Answer from the drawing. Dimensions are ordinates in mm from the lowest x, y and z of the part. A direction names the side the tool comes from. Give positions to 0.01 mm unless a question says otherwise; leave off trailing zeros. Write item = value, one per line.
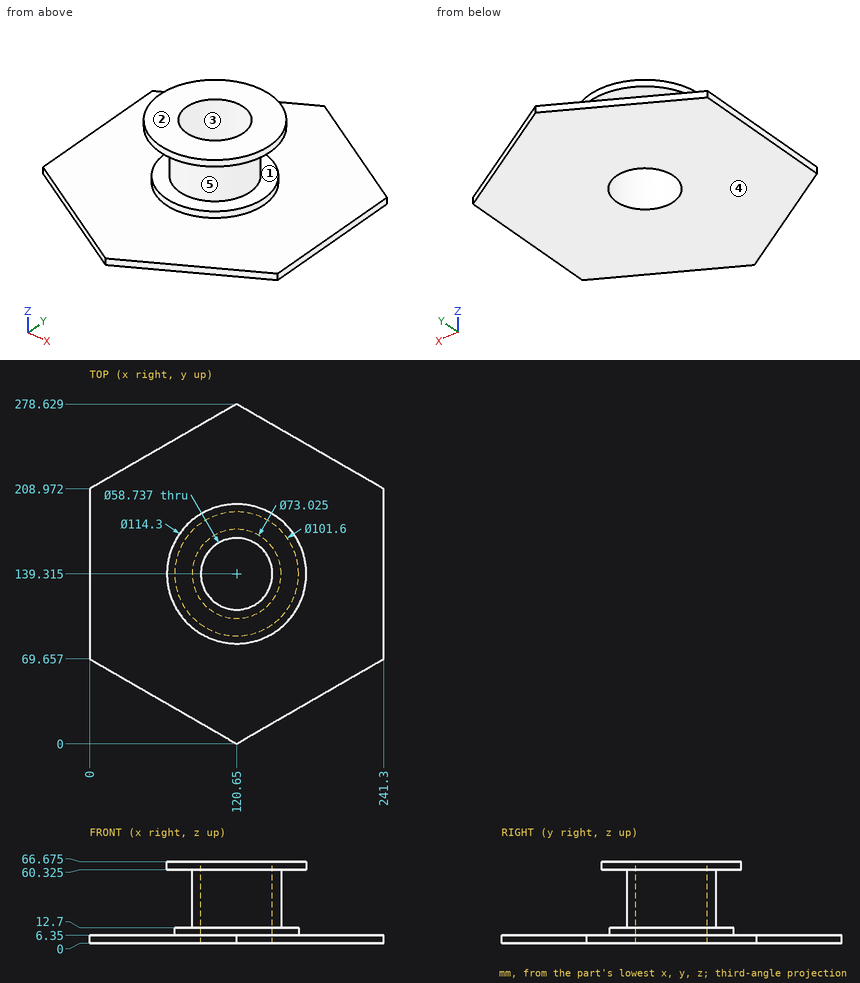
(1) Consider L1, parallel to Z at x = 113.5, y = 183.5 (1 decimal); L2, parallel to Y at x = 120.65, z = 53.5 (1 decimal); L3, parallel to Y at x = 120, z = 34. Determine where each line is inside the solid, lowest interval first.
Checks:
L1 = 0 to 12.7, 60.3 to 66.7
L2 = 102.8 to 109.9, 168.7 to 175.8
L3 = 102.81 to 109.95, 168.68 to 175.82
(2) Given P1, Ø5, axis at y = 143.5, z = 16, coming from the -X side; P2, Ø5, axis at x = 113, y = 247, coming from the +Z side; P3, Ø8, axis at x = 93, z = 25.5, coming from the +Y side; P4, Ø1, axis at x = 42.5, y = 42.5, coming from the +Z side, each flat-ended and moving along its own axis, determine where each tip first touches the part or whether it passes through.
Checks:
P1 = 84.18
P2 = 6.35
P3 = 167.13
P4 = through
(3) A tool of negligible diameter and unlimited length cuts with its end or side. For the marked faces 1 and 2, from which of +Z, -Z, +X, -X, +Y, -Y can it reach the whole face along a straight path? Write none if from no direction.
Checks:
face_1 = none
face_2 = +Z, +X, -X, +Y, -Y
(4) For a pull along Y with two mould halves and no side action, classify the marked faces 3, 4 and 5 as released by +Y, released by -Y, zero draft, split by the parting line, or undercut.
Checks:
face_3 = undercut
face_4 = zero draft
face_5 = split by the parting line
